Geometry check sheet. Reference: the model listing, model coordinates, mm. Coordinates: 2 decimals unless noted, no trailing zeros. Order: outer loops, then holes, each group sorted by start corner. A loop starts at its lowest first (then second) coordinate and runs counter-clockwise, first axis right, second up. Notation, with made-up numbers: (16, 73) -> (32, 73) arc R9 ccw to (32, 89) -> close; hole circle Ø4 at (64, 31.5). An arc over 180 degrees is marked (long way). Answer in a Markdown table with one row per item. Add a question column.
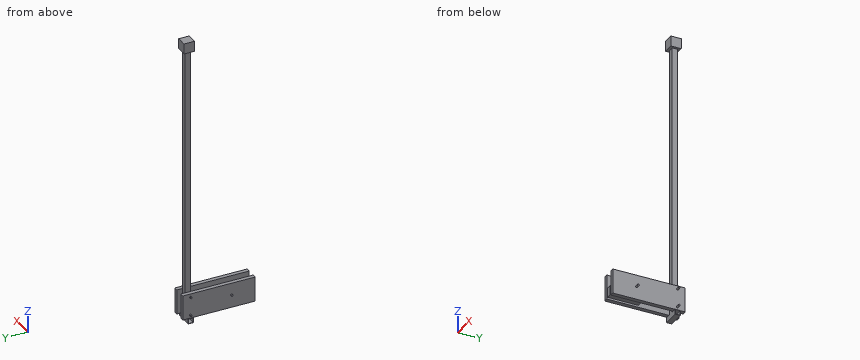
```python
from build123d import *

# Parameters (mm, degrees)
SKETCH013_R   = 9
PAD016_DEPTH  = 200
BOX_W         = 100
BOX_H         = 100
BOX_DEPTH     = 100
SKETCH010_W   = 38.1
SKETCH010_H   = 241.3
PAD013_DEPTH  = 700
SKETCH011_R   = 9
PAD014_DEPTH  = 200
SKETCH014_W   = 50.8
SKETCH014_H   = 50.8
SKETCH014_W_2 = 44.45
SKETCH014_H_2 = 44.45
PAD017_DEPTH  = 160
SKETCH015_W   = 38.1
SKETCH015_H   = 241.3
PAD018_DEPTH  = 700
SKETCH016_W   = 50.8
SKETCH016_H   = 88.9
PAD019_DEPTH  = 300
PAD005_DEPTH  = 3.175
PAD004_DEPTH  = 3.175
PAD002_DEPTH  = 3.175
SKETCH004_R   = 11.675
SKETCH004_R_2 = 8.5
PAD007_DEPTH  = 50.8
SKETCH005_R   = 9
PAD008_DEPTH  = 50.8
SKETCH001_W   = 50.8
SKETCH001_H   = 50.8
SKETCH001_W_2 = 44.45
SKETCH001_H_2 = 44.45
PAD001_DEPTH  = 400
SKETCH006_R   = 11.675
SKETCH006_R_2 = 8.5
PAD009_DEPTH  = 50.8
SKETCH007_R   = 11.675
SKETCH007_R_2 = 8.5
PAD010_DEPTH  = 50.8
SKETCH009_R   = 9
PAD012_DEPTH  = 50.8
SKETCH008_R   = 9
PAD011_DEPTH  = 50.8
SKETCH_W      = 50.8
SKETCH_H      = 50.8
SKETCH_W_2    = 44.45
SKETCH_H_2    = 44.45
PAD_DEPTH     = 2650
PAD006_DEPTH  = 3.175
SKETCH012_R   = 9
PAD015_DEPTH  = 200


with BuildPart() as lower_bolt:
    # Sketch013 → Pad016 (new body)
    with BuildSketch(Plane(origin=(-65, 25.4, 30), x_dir=(0, 0, -1), z_dir=(1, 0, 0))):
        Circle(SKETCH013_R)
    extrude(amount=PAD016_DEPTH)


with BuildPart() as cube:
    # Box → Box (new body)
    with BuildSketch(Plane(origin=(-25, -25, 2650), x_dir=(1, 0, 0), z_dir=(0, 0, 1))):
        with Locations((50, 50)):
            Rectangle(BOX_W, BOX_H)
    extrude(amount=BOX_DEPTH)


with BuildPart() as joist:
    # Sketch010 → Pad013 (new body)
    with BuildSketch(Plane(origin=(-50.8, 100, 0), x_dir=(1, 0, 0), z_dir=(0, -1, 0))):
        with Locations((19.05, 120.65)):
            Rectangle(SKETCH010_W, SKETCH010_H)
    extrude(amount=PAD013_DEPTH)


with BuildPart() as brace_bolt:
    # Sketch011 → Pad014 (new body)
    with BuildSketch(Plane(origin=(-65, -370, 125.4), x_dir=(0, 0, -1), z_dir=(1, 0, 0))):
        Circle(SKETCH011_R)
    extrude(amount=PAD014_DEPTH)


with BuildPart() as lower_support_tube:
    # Sketch014 → Pad017 (new body)
    with BuildSketch(Plane(origin=(105, 0, 0), x_dir=(0, 0, -1), z_dir=(1, 0, 0))):
        with Locations((25.4, 25.4)):
            Rectangle(SKETCH014_W, SKETCH014_H)
        with Locations((25.4, 25.4)):
            Rectangle(SKETCH014_W_2, SKETCH014_H_2, mode=Mode.SUBTRACT)
    extrude(amount=-PAD017_DEPTH)


with BuildPart() as pad018:
    # Sketch015 → Pad018 (new body)
    with BuildSketch(Plane(origin=(62.8, 100, 0), x_dir=(1, 0, 0), z_dir=(0, -1, 0))):
        with Locations((19.05, 120.65)):
            Rectangle(SKETCH015_W, SKETCH015_H)
    extrude(amount=PAD018_DEPTH)


with BuildPart() as brace_support:
    # Sketch016 → Pad019 (new body)
    with BuildSketch(Plane(origin=(0, -300, 11.1), x_dir=(1, 0, 0), z_dir=(0, -1, 0))):
        with Locations((25.4, 44.45)):
            Rectangle(SKETCH016_W, SKETCH016_H)
    extrude(amount=PAD019_DEPTH)


with BuildPart() as gusset3:
    # Sketch003 → Pad005 (new body)
    with BuildSketch(Plane(origin=(47.625, 0, 150.8), x_dir=(0, 1, 0), z_dir=(1, 0, 0))):
        with BuildLine():
            Line((0, 0), (0, 50))
            ThreePointArc((-50, 0), (-15.471731, 15.471731), (0, 50))
            Line((0, 0), (-50, 0))
        make_face()
    extrude(amount=PAD005_DEPTH)


with BuildPart() as gusset2:
    # MirroredSketch → Pad004 (new body)
    with BuildSketch(Plane(origin=(0, 0, 100), x_dir=(0, 1, 0), z_dir=(1, 0, 0))):
        with BuildLine():
            Line((0, 0), (0, -50))
            ThreePointArc((0, -50), (-15.471731, -15.471731), (-50, 0))
            Line((0, 0), (-50, 0))
        make_face()
    extrude(amount=PAD004_DEPTH)


with BuildPart() as gusset1:
    # Sketch002 → Pad002 (new body)
    with BuildSketch(Plane(origin=(0, 0, 150.8), x_dir=(0, 1, 0), z_dir=(1, 0, 0))):
        with BuildLine():
            Line((0, 0), (0, 50))
            ThreePointArc((-50, 0), (-15.471731, 15.471731), (0, 50))
            Line((0, 0), (-50, 0))
        make_face()
    extrude(amount=PAD002_DEPTH)


with BuildPart() as brace_bolt_tube:
    # Sketch004 → Pad007 (new body)
    with BuildSketch(Plane(origin=(0, -370, 125.4), x_dir=(0, 0, -1), z_dir=(1, 0, 0))):
        Circle(SKETCH004_R)
        Circle(SKETCH004_R_2, mode=Mode.SUBTRACT)
    extrude(amount=PAD007_DEPTH)


with BuildPart() as brace_bolt_hole:
    # Sketch005 → Pad008 (new body)
    with BuildSketch(Plane(origin=(0, -370, 125.4), x_dir=(0, 0, -1), z_dir=(1, 0, 0))):
        Circle(SKETCH005_R)
    extrude(amount=PAD008_DEPTH)


with BuildPart() as brace_fusion:
    # Sketch001 → Pad001 (new body)
    with BuildSketch(Plane(origin=(0, 0, 100), x_dir=(1, 0, 0), z_dir=(0, -1, 0))):
        with Locations((25.4, 25.4)):
            Rectangle(SKETCH001_W, SKETCH001_H)
        with Locations((25.4, 25.4)):
            Rectangle(SKETCH001_W_2, SKETCH001_H_2, mode=Mode.SUBTRACT)
    extrude(amount=PAD001_DEPTH)

    # Cut: cut Brace Bolt Hole
    add(brace_bolt_hole.part, mode=Mode.SUBTRACT)

    # Fusion: union Brace Bolt Tube
    add(brace_bolt_tube.part)


with BuildPart() as lower_bolt_tube:
    # Sketch006 → Pad009 (new body)
    with BuildSketch(Plane(origin=(0, 25.4, 30), x_dir=(0, 0, -1), z_dir=(1, 0, 0))):
        Circle(SKETCH006_R)
        Circle(SKETCH006_R_2, mode=Mode.SUBTRACT)
    extrude(amount=PAD009_DEPTH)


with BuildPart() as upper_bolt_tube:
    # Sketch007 → Pad010 (new body)
    with BuildSketch(Plane(origin=(0, 25.4, 210), x_dir=(0, 0, -1), z_dir=(1, 0, 0))):
        Circle(SKETCH007_R)
        Circle(SKETCH007_R_2, mode=Mode.SUBTRACT)
    extrude(amount=PAD010_DEPTH)


with BuildPart() as upper_bolt_hole:
    # Sketch009 → Pad012 (new body)
    with BuildSketch(Plane(origin=(0, 25.4, 210), x_dir=(0, 0, -1), z_dir=(1, 0, 0))):
        Circle(SKETCH009_R)
    extrude(amount=PAD012_DEPTH)


with BuildPart() as lower_bolt_hole:
    # Sketch008 → Pad011 (new body)
    with BuildSketch(Plane(origin=(0, 25.4, 30), x_dir=(0, 0, -1), z_dir=(1, 0, 0))):
        Circle(SKETCH008_R)
    extrude(amount=PAD011_DEPTH)


with BuildPart() as post_fusion:
    # Sketch → Pad (new body)
    with BuildSketch(Plane.XY):
        with Locations((25.4, 25.4)):
            Rectangle(SKETCH_W, SKETCH_H)
        with Locations((25.4, 25.4)):
            Rectangle(SKETCH_W_2, SKETCH_H_2, mode=Mode.SUBTRACT)
    extrude(amount=PAD_DEPTH)

    # Cut001: cut Lower Bolt Hole
    add(lower_bolt_hole.part, mode=Mode.SUBTRACT)

    # Cut002: cut Upper Bolt Hole
    add(upper_bolt_hole.part, mode=Mode.SUBTRACT)

    # Fusion001: union Lower Bolt Tube, Upper Bolt Tube
    add(lower_bolt_tube.part)
    add(upper_bolt_tube.part)


with BuildPart() as fusion004:
    # MirroredSketch001 → Pad006 (new body)
    with BuildSketch(Plane(origin=(47.625, 0, 100), x_dir=(0, 1, 0), z_dir=(1, 0, 0))):
        with BuildLine():
            Line((0, 0), (0, -50))
            ThreePointArc((0, -50), (-15.471731, -15.471731), (-50, 0))
            Line((0, 0), (-50, 0))
        make_face()
    extrude(amount=PAD006_DEPTH)

    # Fusion002: union Gusset3, Gusset2, Gusset1, Brace Fusion, Post Fusion
    add(gusset3.part)
    add(gusset2.part)
    add(gusset1.part)
    add(brace_fusion.part)
    add(post_fusion.part)

    # Fusion003: union Joist, Brace Bolt, Lower support Tube, Pad018, Brace Support
    add(joist.part)
    add(brace_bolt.part)
    add(lower_support_tube.part)
    add(pad018.part)
    add(brace_support.part)

    # Fusion004: union Cube
    add(cube.part)


with BuildPart() as fusion005:
    # Sketch012 → Pad015 (new body)
    with BuildSketch(Plane(origin=(-65, 25.4, 210), x_dir=(0, 0, -1), z_dir=(1, 0, 0))):
        Circle(SKETCH012_R)
    extrude(amount=PAD015_DEPTH)

    # Fusion005: union Lower Bolt, Fusion004
    add(lower_bolt.part)
    add(fusion004.part)


solid = fusion005.part
```
(1) Scan lines: line 1 along Z through (x, y) = (-24, 23.5) (3 decimals); line 2 along X through (y, z) = (-273.5, 131) (3 decimals); line 3 along X through (y, z) = (23, 2485) (3 decimals). Record each from-to range of solid material in increasing order.
(2) Go/stop test with flat-tipped pins: P1, Ø13.5, axis at x = 15.5, z = 799.5, coming from the +Y side; P2, Ø13.5, axis at y = 18.5, z = 1307.5, coming from the -X side; P3, Ø12, axis at x = 90, y = -493, coming from the +Z side. Record where each tip stops, or that it passes through.
(3) Cross-section at B-B (z = 2056.5). Enter the section's corners in (x, y) (3 decimals).
(4) Cross-section at A-A (y = -513). Enter the section's corners in (x, z), plus the area to 3 significant figures.
Checks:
| question | item | result |
|---|---|---|
| 1 | line 1 | -50.8 to -47.625, -3.175 to 241.3, 2650 to 2750 |
| 1 | line 2 | -50.8 to -12.7, 0 to 3.175, 47.625 to 50.8, 62.8 to 100.9 |
| 1 | line 3 | 0 to 3.175, 47.625 to 50.8 |
| 2 | P1 | y = 50.8 |
| 2 | P2 | x = 0 |
| 2 | P3 | z = 241.3 |
| 3 | outline | (0, 0) -> (50.8, 0) -> (50.8, 50.8) -> (0, 50.8) -> close; hole (3.175, 3.175) -> (47.625, 3.175) -> (47.625, 47.625) -> (3.175, 47.625) -> close |
| 4 | outline | (-50.8, 0) -> (-12.7, 0) -> (-12.7, 241.3) -> (-50.8, 241.3) -> close; (0, 11.1) -> (50.8, 11.1) -> (50.8, 100) -> (0, 100) -> close; (62.8, 0) -> (100.9, 0) -> (100.9, 241.3) -> (62.8, 241.3) -> close |
| 4 | area | 22,900 mm² |
